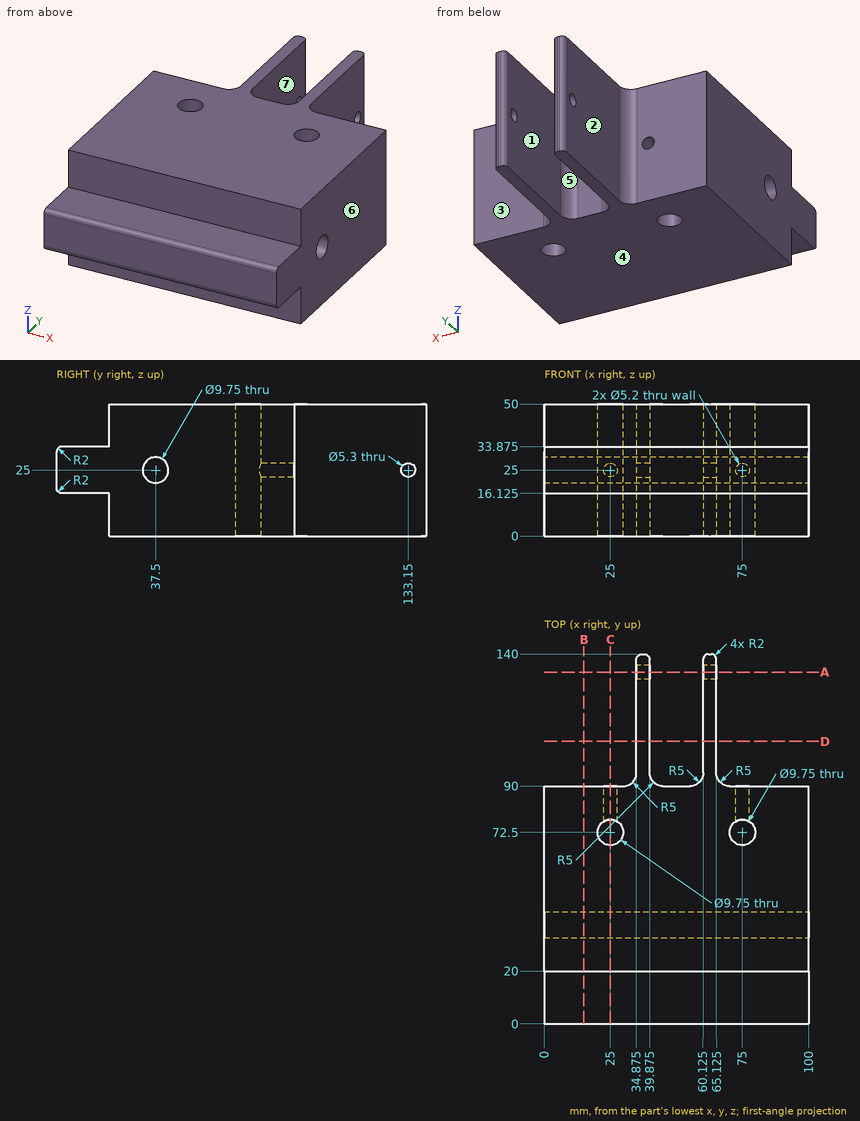
Study the drawing (mm; zero at the part's minimum x, y, z) and answer. A direction names the side the tool comes from. Round coordinates to 2 decimals unless told otherwise and drop trailing zeros. Loops run counter-clockwise (first coordinate to the right, second up) from the corner with the lowest first, then second, coordinate; pieces in that order, holes last. Notation, with made-up numbers: (15.25, -30.5) - (74.25, -30.5) arc R20 cw to (74.25, -13.5) - close; hole circle Ø1 at (19, 72.25). An arc over 180 degrees is marked (long way). Use one line per item in the form item = value. Start each with the question number.
1. The part is cut by section D-D on y = 107. Determine the outline of the cut face in (x, z) (3 decimals), then the cut area to 3 significant figures.
2. The part is cut by section A-A on y = 133.15. Determine the outline of the cut face in (x, z) (3 decimals), then the cut area to 3 significant figures.
3. The part is cut by section B-B on x = 15. Determine the outline of the cut face in (y, z) (3 decimals).
4. Consider line 1 (X direction, y = 72.5, z = 22) (3 decimals); line 2 (X direction, y = 72, z = 21); line 3 (Z direction, x = 63.25, y = 133.15). Determine where each line is inside the solid, lowest interval first. Write a range as [from, to].
5. For a pull along X with two mould halves and no side action, classify the marked faces 4, 5, 6 and 7 as pulls with the +X half, pulls with the -X half, needs draft (parallel to the pull), parting line crosses it, or undercut.
6. Given pin 1 Ø6 at (x, y) = (25, 72.5) entering from +Z; pin 2 Ø6 at (x, z) = (75, 25) entering from +Y; pin 3 Ø21.5 at (y, z) = (120, 34.5) entering from +X (3 decimals); pin 4 Ø6 at (y, z) = (133.15, 25) entering from -X (3 decimals), each flat-ended and moving along its own axis, determine where each tip first touches the part or whether it passes through.
7. A tool of negligible diameter and unlimited length cuts with its end or side. For the marked faces 1, 2 and 3, from which of +Z, -Z, +X, -X, +Y, -Y can it reach the whole face along a straight path? Write none if from no direction.
8. The part is cut by section C-C on x = 25. Determine the outline of the cut face in (y, z) (3 decimals).
Geometry check:
q1.outline = (34.875, 0) - (39.875, 0) - (39.875, 50) - (34.875, 50) - close; (60.125, 0) - (65.125, 0) - (65.125, 50) - (60.125, 50) - close
q1.area = 500 mm^2
q2.outline = (34.875, 0) - (39.875, 0) - (39.875, 22.35) - (34.875, 22.35) - close; (34.875, 27.65) - (39.875, 27.65) - (39.875, 50) - (34.875, 50) - close; (60.125, 0) - (65.125, 0) - (65.125, 22.35) - (60.125, 22.35) - close; (60.125, 27.65) - (65.125, 27.65) - (65.125, 50) - (60.125, 50) - close
q2.area = 447 mm^2
q3.outline = (0, 18.125) arc R2 ccw to (2, 16.125) - (20, 16.125) - (20, 0) - (90, 0) - (90, 50) - (20, 50) - (20, 33.875) - (2, 33.875) arc R2 ccw to (0, 31.875) - close; hole circle Ø9.75 at (37.5, 25)
q4.line_1 = [0, 20.125], [29.875, 70.125], [79.875, 100]
q4.line_2 = [0, 20.15], [29.85, 70.15], [79.85, 100]
q4.line_3 = [0, 22.35], [27.65, 50]
q5.face_4 = needs draft
q5.face_5 = undercut
q5.face_6 = pulls with the +X half
q5.face_7 = undercut
q6.pin_1 = through
q6.pin_2 = 90
q6.pin_3 = 65.125
q6.pin_4 = 34.875
q7.face_1 = +Z, -Z, +Y
q7.face_2 = +Z, -Z, -X, +Y
q7.face_3 = +Z, -Z, +X, +Y
q8.outline = (0, 18.125) arc R2 ccw to (2, 16.125) - (20, 16.125) - (20, 0) - (67.625, 0) - (67.625, 50) - (20, 50) - (20, 33.875) - (2, 33.875) arc R2 ccw to (0, 31.875) - close; (77.375, 0) - (90, 0) - (90, 22.4) - (77.375, 22.4) - close; (77.375, 27.6) - (90, 27.6) - (90, 50) - (77.375, 50) - close; hole circle Ø9.75 at (37.5, 25)
